Work out the finished part from the listing and answer in its coordinate system (mm). Face numbers are marked on the shaded views. A direction names the side the tool comes from. Give positions to 0.01 mm unless a question says otherwise; leave off trailing zeros. Write each loop counter-clockwise with the first axis right and the second up, starting at its lowest first coordinate (ties: lowest second). Pieces come first, ordered by that corner, then holes. Notation, with made-up numbers: (20, 38) -> (64, 38) arc R15 cw to (64, 65) -> close; hole circle Ø8 at (5.5, 3). An arc over 180 degrees is marked (long way). Use a Markdown table: item, result. Add a question column.
Q1. Section A-A, the plane z = 199 is taken. Give the vertices of the cut face in (x, y), plus the area to 3 significant figures.
Q2. For the marked faces 1, 2, 3 and 4, determine the directions among +Z, -Z, +X, -X, +Y, -Y from which every point of the face is accessible in a straight line to the end or side of a thin tool.
Q3. Consider line 1 (Z direction, x = -34.5, y = 42); line 2 (X direction, y = 11.5, z = 135); line 3 (Z direction, x = -12.5, y = -11.5). Determine where each line is inside the solid, lowest interval first.
Q4. Section B-B, the plane y = 50.5 is taken. Give the vertices of the cut face in (x, z), plus the area to 3 significant figures.
Q5. Section C-C, the plane z = -69.5 is taken. Give the vertices of the cut face in (x, y), plus the area to 3 significant figures.
Q6. Each of these flat-tipped pins is pushed along its axis until it touches: pin 1 Ø12 at (x, y) = (22.5, 22.5) entering from -Z; pin 2 Ø9.5 at (y, z) = (-7, 96) entering from -X; pin 3 Ø6 at (y, z) = (42, 62) entering from -X. Where does it stop, or does it pass through?
from build123d import *

# Parameters (mm, degrees)
F0_R         = 63.5
F1_DEPTH     = 9.398
F2_R         = 38.1
F3_DEPTH     = 111.506
F4_W         = 35.051997751
F4_H         = 81.7880034447
F5_DEPTH     = 304.8
F6_R         = 24.5284097937
F7_T1_DEPTH  = 296.3349893283
F8_T1_DEPTH  = 227.6667963807
F8_T3_DEPTH  = 227.6667963807
F9_T1_DEPTH  = 194.6467963807
F9_T3_DEPTH  = 194.6467963807
F10_T1_DEPTH = 270.8026681705


# Not quite as in the source:
# - a fillet or chamfer that OpenCascade refuses, or shapes differently, is made with other operations: its cross-section is extruded or revolved along the edge and cut away or added


with BuildPart() as f1:
    # F0 (on Top) → F1 (new body)
    with BuildSketch(Plane.XY):
        Circle(F0_R)
    extrude(amount=F1_DEPTH)

    # F2 (on face) → F3 (join)
    with BuildSketch(Plane(origin=(0, 0, 0), x_dir=(1, 0, 0), z_dir=(0, 0, -1))):
        Circle(F2_R)
    extrude(amount=F3_DEPTH)

    # F4 (on face) → F5 (join)
    with BuildSketch(Plane.XY.offset(9.398)):
        Rectangle(F4_W, F4_H)
    extrude(amount=F5_DEPTH)

    # F6
    f6_edges = [f1.edges().sort_by_distance(p)[0] for p in [
        (-38.1, 0, -111.506),
    ]]
    fillet(f6_edges, radius=F6_R)

    # F7: chamfer of 50.8 on 2 edges, made by hand

    # F7_s2 → F7_t1 (cut)
    with BuildSketch(Plane.YZ.offset(-148.1674946642)):
        Polygon((40.8940017223, 263.398), (-9.9059982777, 314.198), (40.8940017223, 314.198), align=None)
        Polygon((-40.8940017223, 263.398), (9.9059982777, 314.198), (-40.8940017223, 314.198), align=None)
    extrude(amount=F7_T1_DEPTH, mode=Mode.SUBTRACT)

    # F8: chamfer of 33.02 on 2 edges, made by hand

    # F8_s2 → F8_t1 (cut)
    with BuildSketch(Plane(origin=(0, -51.2066322141, 51.2066322141), x_dir=(1, 0, 0), z_dir=(0, -0.7071067812, 0.7071067812))):
        Polygon((17.5259988755, 182.1469378787), (-15.4940011245, 215.1669378787), (17.5259988755, 215.1669378787), align=None)
    extrude(amount=F8_T1_DEPTH, mode=Mode.SUBTRACT)

    # F8_s4 → F8_t3 (cut)
    with BuildSketch(Plane(origin=(0, -212.1913677859, 212.1913677859), x_dir=(1, 0, 0), z_dir=(0, 0.7071067812, -0.7071067812))):
        Polygon((-17.5259988755, -182.1469378787), (15.4940011245, -215.1669378787), (-17.5259988755, -215.1669378787), align=None)
    extrude(amount=F8_T3_DEPTH, mode=Mode.SUBTRACT)

    # F9: chamfer of 33.02 on 2 edges, made by hand

    # F9_s2 → F9_t1 (cut)
    with BuildSketch(Plane(origin=(0, 188.8427018711, 188.8427018711), x_dir=(1, 0, 0), z_dir=(0, -0.7071067812, -0.7071067812))):
        Polygon((-17.5259988755, 182.1469378787), (15.4940011245, 215.1669378787), (-17.5259988755, 215.1669378787), align=None)
    extrude(amount=F9_T1_DEPTH, mode=Mode.SUBTRACT)

    # F9_s4 → F9_t3 (cut)
    with BuildSketch(Plane(origin=(0, 51.2066322141, 51.2066322141), x_dir=(1, 0, 0), z_dir=(0, 0.7071067812, 0.7071067812))):
        Polygon((17.5259988755, -182.1469378787), (-15.4940011245, -215.1669378787), (17.5259988755, -215.1669378787), align=None)
    extrude(amount=F9_T3_DEPTH, mode=Mode.SUBTRACT)

    # F10: fillet of radius 25.4 on 4 edges, made by hand

    # F10_s2 → F10_t1 (cut)
    with BuildSketch(Plane.XY.offset(9.398)):
        with BuildLine():
            ThreePointArc((7.8740011245, 40.8940017223), (-10.0865111176, 33.4545139645), (-17.5259988755, 15.4940017223))
            Line((-17.5259988755, 15.4940017223), (-17.5259988755, 40.8940017223))
            Line((-17.5259988755, 40.8940017223), (7.8740011245, 40.8940017223))
        make_face()
        with BuildLine():
            ThreePointArc((17.5259988755, 15.4940017223), (10.0865111176, 33.4545139645), (-7.8740011245, 40.8940017223))
            Line((-7.8740011245, 40.8940017223), (17.5259988755, 40.8940017223))
            Line((17.5259988755, 40.8940017223), (17.5259988755, 15.4940017223))
        make_face()
        with BuildLine():
            ThreePointArc((-17.5259988755, -15.4940017223), (-10.0865111176, -33.4545139645), (7.8740011245, -40.8940017223))
            Line((7.8740011245, -40.8940017223), (-17.5259988755, -40.8940017223))
            Line((-17.5259988755, -40.8940017223), (-17.5259988755, -15.4940017223))
        make_face()
        with BuildLine():
            ThreePointArc((17.5259988755, -15.4940017223), (10.0865111176, -33.4545139645), (-7.8740011245, -40.8940017223))
            Line((-7.8740011245, -40.8940017223), (17.5259988755, -40.8940017223))
            Line((17.5259988755, -40.8940017223), (17.5259988755, -15.4940017223))
        make_face()
    extrude(amount=F10_T1_DEPTH, mode=Mode.SUBTRACT)


solid = f1.part
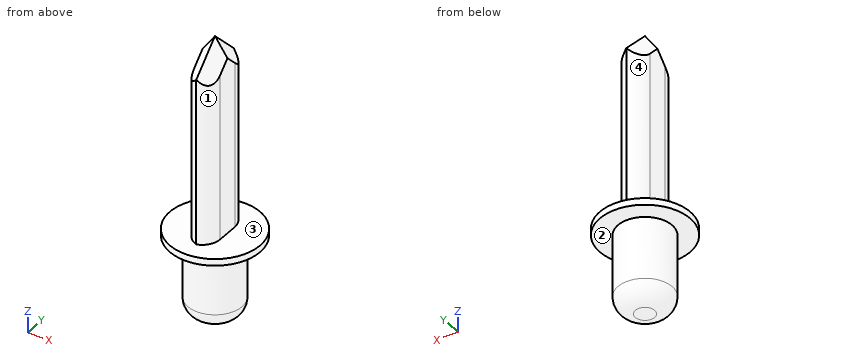
Result set:
| question | item | result |
|---|---|---|
| 1 | outline | (-17.53, -15.49) arc R25.4 ccw to (0, -39.64) arc R25.4 ccw to (17.53, -15.49) -> (17.53, 15.49) arc R25.4 ccw to (0, 39.64) arc R25.4 ccw to (-17.53, 15.49) -> close |
| 1 | area | 2,330 mm2 |
| 2 | face 1 | +Z, +X, -Y |
| 2 | face 2 | -Z |
| 2 | face 3 | +Z |
| 2 | face 4 | +Z, -X, +Y |
| 3 | line 1 | z = 0 to 9.4 |
| 3 | line 2 | x = -17.53 to 17.53 |
| 3 | line 3 | z = -111.27 to 253.2 |
| 4 | outline | (-38.5, 0) -> (38.5, 0) -> (38.5, 9.4) -> (-38.5, 9.4) -> close |
| 4 | area | 724 mm2 |
| 5 | outline | circle Ø76.2 at (0, 0) |
| 5 | area | 4,560 mm2 |
| 6 | pin 1 | stops at z = -108.23 |
| 6 | pin 2 | stops at x = -17.53 |
| 6 | pin 3 | stops at x = -1.75 |
